Could you check a few things on this model? Use its own coordinates, in mm. Give positions to 0.01 mm unless a question says otherwise; leave off trailing zeros. Write each loop counter-clockwise with the first axis right and the second up, starting at its lowest first coordinate (ties: lowest second). Pieces come first, ordered by that corner, then holes. Notation, with made-up numbers: (-35, 57.5) - (12, 57.5) arc R15 ccw to (12, 82.5) - close; hole circle Ø9 at (14.25, 48.25). An arc over 180 degrees is marked (long way). Answer as CSV lines item,"result". Start each with the question number.
Q1. Imagine slicing it at B-B on z = -35. List the corners of the cut face in (x, y) for me, and give its area (3 significant figures).
Q2. Imagine slicing it at A-A on x = -50. List the corners of the cut face in (y, z) for me, and give its area (3 significant figures).
Q3. If I drill on line 1 along Z through (x, y) = (50, 4.6); line 2 along Z through (x, y) = (47.5, 5.55); line 3 along X through (y, z) = (2.1, 33), over which ranges is the centre line in solid material (lowest first)?
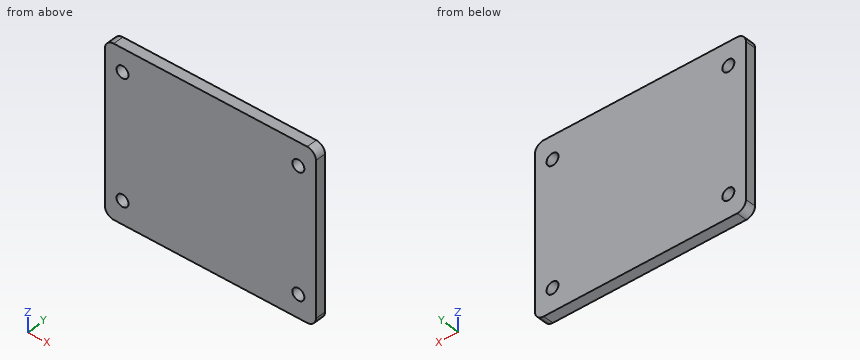
Autodesk Inventor part; units mm, degrees
ref_plane "YZ Plane" through (0, 0, 0) normal (1, 0, 0) x (0, 1, 0)
ref_plane "XZ Plane" through (0, 0, 0) normal (0, 1, 0) x (-1, 0, 0)
ref_plane "XY Plane" through (0, 0, 0) normal (0, 0, 1) x (1, 0, 0)
sketch "Sketch1" plane through (0, 0, 0) normal (0, 1, 0) x (-1, 0, 0)
  line L0 (55, -48) -> (-55, -48)
  line L1 (-60, -43) -> (-60, 43)
  line L2 (-55, 48) -> (55, 48)
  line L3 (60, 43) -> (60, -43)
  line L4 (50, -35) -> (-50, -35) construction
  line L5 (-50, -35) -> (-50, 35) construction
  line L6 (-50, 35) -> (50, 35) construction
  line L7 (50, 35) -> (50, -35) construction
  arc A0 (60, 43) -> (55, 48) centre (55, 43) ccw
  arc A1 (-55, 48) -> (-60, 43) centre (-55, 43) ccw
  arc A2 (-60, -43) -> (-55, -48) centre (-55, -43) ccw
  arc A3 (55, -48) -> (60, -43) centre (55, -43) ccw
  circle A4 centre (50, -35) radius 3.4
  circle A5 centre (50, 35) radius 3.4
  circle A6 centre (-50, -35) radius 3.4
  circle A7 centre (-50, 35) radius 3.4
  line L8 (0, -20) -> (0, 20) construction
  line L9 (25, -20) -> (25, 20) construction
  line L10 (-25, 20) -> (-25, -20) construction
  arc A8 (-25, -20) -> (25, -20) centre (0, -20) ccw construction
  arc A9 (25, 20) -> (-25, 20) centre (0, 20) ccw construction
  point P0 (0, 0)
  point P1 (-60, 0)
  point P2 (0, -48)
  point P3 (0, -35)
  point P4 (-50, 0)
  point P5 (0, 0)
  dimension "d0" = 96
  dimension "d1" = 120
  dimension "d2" = 70
  dimension "d3" = 100
  dimension "d4" = 5
  dimension "d5" = 6.8
  dimension "d6" = 6.8
  dimension "d8" = 6.8
  dimension "d10" = 6.8
  dimension "d13" = 25
  dimension "d14" = 40
extrude "Extrusion1" add sketch "Sketch1" along normal blind 6
equation "\"d0\" = moduleHeight"
equation "\"d1\" = moduleWidth"
equation "\"d2\" = moduleMountH"
equation "\"d3\" = moduleMountW"
equation "\"d4\" = moduleCornerR"
equation "\"d5\" = moduleMountD"
equation "\"d6\" = moduleMountD"
equation "\"d8\" = moduleMountD"
equation "\"d10\" = moduleMountD"
equation "\"d13\" = moduleOpeningR"
equation "\"d14\" = moduleOpeningH"
equation "\"d15\" = thickness"
equation "\"moduleWidth\" = 120"
equation "\"moduleHeight\" = 96"
equation "\"moduleMountW\" = 100"
equation "\"moduleMountH\" = 70"
equation "\"moduleMountD\" = 6.8"
equation "\"moduleCornerR\" = 5"
equation "\"moduleOpeningR\" = 25"
equation "\"moduleOpeningH\" = 40"
equation "\"thickness\" = 6"
properties part number "Module_base"
Conclusion:
1,outline,"(-60, 0) - (-53.4, 0) - (-53.4, 6) - (-60, 6) - close; (-46.6, 0) - (46.6, 0) - (46.6, 6) - (-46.6, 6) - close; (53.4, 0) - (60, 0) - (60, 6) - (53.4, 6) - close"
1,area,"638 mm^2"
2,outline,"(0, -48) - (6, -48) - (6, -38.4) - (0, -38.4) - close; (0, -31.6) - (6, -31.6) - (6, 31.6) - (0, 31.6) - close; (0, 38.4) - (6, 38.4) - (6, 48) - (0, 48) - close"
2,area,"494 mm^2"
3,line 1,"-48 to -38.4, -31.6 to 31.6, 38.4 to 48"
3,line 2,"-48 to -37.3, -32.7 to 32.7, 37.3 to 48"
3,line 3,"-60 to -52.75, -47.25 to 47.25, 52.75 to 60"
